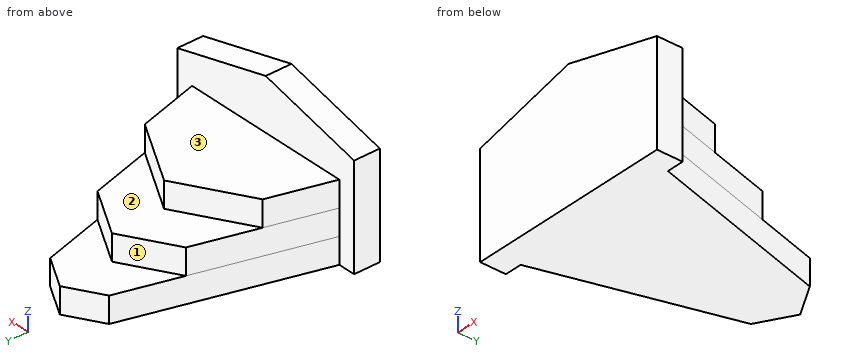
from build123d import *

# Parameters (mm, degrees)
EXTRUDE1_DEPTH = 15
EXTRUDE2_DEPTH = 15
EXTRUDE3_DEPTH = 15
EXTRUDE4_DEPTH = 15


with BuildPart() as part:
    # Sketch1 → Extrude1 (new body)
    with BuildSketch(Plane(origin=(0, 0, 0), x_dir=(1, 0, 0), z_dir=(0, 1, 0))):
        Polygon((0, 0), (-60, -15), (-120, 0), (-120, 60), (0, 60), align=None)
    extrude(amount=EXTRUDE1_DEPTH)

    # Sketch2 → Extrude2 (add)
    with BuildSketch(Plane(origin=(0, 0, -60), x_dir=(-1, 0, 0), z_dir=(0, 0, -1))):
        Polygon((110, 15), (80, 123.452994616), (60, 135), (40, 123.452994616), (10, 15), align=None)
    extrude(amount=-EXTRUDE2_DEPTH)

    # Sketch3 → Extrude3 (add)
    with BuildSketch(Plane.XY.offset(-45)):
        Polygon((-10, 15), (-30, 87.301996411), (-60, 104.622504486), (-90, 87.301996411), (-110, 15), align=None)
    extrude(amount=EXTRUDE3_DEPTH)

    # Sketch4 → Extrude4 (add)
    with BuildSketch(Plane.XY.offset(-30)):
        Polygon((-110, 15), (-10, 15), (-20, 51.150998205), (-60, 74.245008973), (-100, 51.150998205), align=None)
    extrude(amount=EXTRUDE4_DEPTH)


solid = part.part
For this review, take the finished solid that the model builds, in its own axes (mm). Face numbers are marked on the shaded views. A direction names the side the tool comes from. Coordinates: 2 decimals unless noted, no trailing zeros. Order: outer loops, then holes, each group sorted by start corner. A loop starts at its lowest first (then second) coordinate and runs counter-clockwise, first axis right, second up. Notation, with made-up numbers: (88.5, 76.25) - (95.5, 76.25) arc R29 cw to (95.5, 99.25) - close; hole circle Ø3 at (77, 18). An arc over 180 degrees is marked (long way). Answer as CSV lines item,"result". Start each with the question number.
1) Add section A-A (z = -47.5). State the section outline as (x, y) points.
2) Machinability: for the marked faces 1, 2 and 3, which of the approach directions +Z, -Z, +X, -X, +Y, -Y give a long, thin tool a straight path to every point of the face, cutting with its end or side? Answer none if there is none.
3) To check wall thickness, follow line 1 along Y through (x, z) = (-24, -0.5); line 2 along Z through (x, y) = (-56.5, 88); line 3 along Z through (x, y) = (-71.5, 38.5). State the ranges of each line that lie inside material, in increasing order. Write a range as [from, to].
4) Add section B-B (y = 64). State the section outline as (x, z) points, then the cut area to 3 significant figures.
5) Add section D-D (z = -36). State the section outline as (x, y) points.
6) Insertion check: P1, Ø4, axis at x = -107.5, z = 0.5, coming from the +Y side; P2, Ø12, axis at y = 68, z = -29, coming from the +X side; P3, Ø1, axis at x = -81, y = 63.5, coming from the +Z side. Each pin has a flat end and moves straight along its axis. Give the tip position at first contact, or say it passes through.
7) Add section C-C (x = -56). State the section outline as (y, z) points, then the cut area to 3 significant figures.
Result:
1,outline,"(-120, 0) - (0, 0) - (0, 15) - (-10, 15) - (-40, 123.45) - (-60, 135) - (-80, 123.45) - (-110, 15) - (-120, 15) - close"
2,face 1,"+Z, -X, +Y"
2,face 2,"+Z, +Y"
2,face 3,"+Z, +X, -X, +Y"
3,line 1,"[0, 15]"
3,line 2,"[-60, -30]"
3,line 3,"[-60, -15]"
4,outline,"(-96.45, -60) - (-23.55, -60) - (-23.55, -30) - (-42.26, -30) - (-42.26, -15) - (-77.74, -15) - (-77.74, -30) - (-96.45, -30) - close"
4,area,"2,720 mm^2"
5,outline,"(-120, 0) - (0, 0) - (0, 15) - (-10, 15) - (-30, 87.3) - (-60, 104.62) - (-90, 87.3) - (-110, 15) - (-120, 15) - close"
6,P1,"y = 15"
6,P2,"x = -23.02"
6,P3,"z = -30"
7,outline,"(0, -60) - (132.69, -60) - (132.69, -45) - (102.31, -45) - (102.31, -30) - (71.94, -30) - (71.94, -15) - (15, -15) - (15, 14) - (0, 14) - close"
7,area,"5,040 mm^2"
